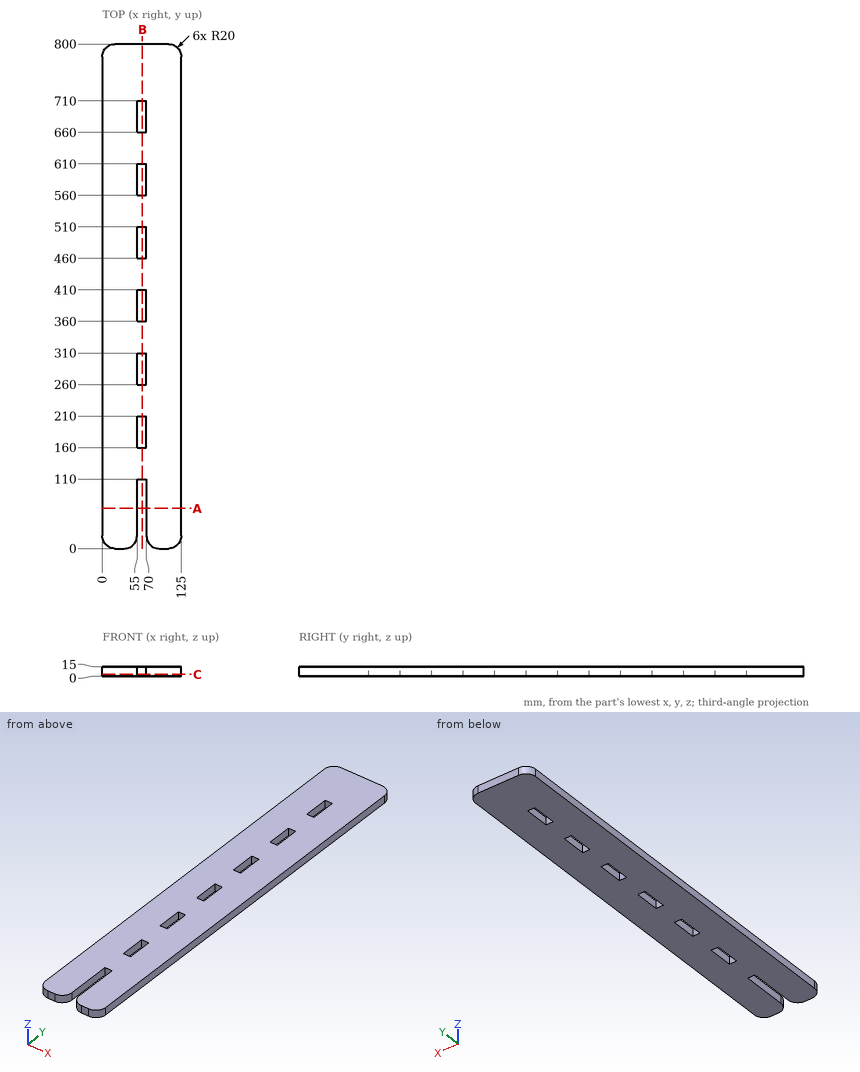
Design review of the part shown in the three views and the two pictorial views. Dimensions are in mm from the part's minimum x, y and z. Round coordinates to 2 decimals unless told otherwise and drop trailing zeros. Write each loop counter-clockwise with the first axis right and the second up, starting at its lowest first coordinate (ties: lowest second). Pieces come first, ordered by that corner, then holes. Notation, with made-up numbers: (-36.5, 12.25) -> (-29.5, 12.25) arc R16 cw to (-29.5, 20.25) -> close; hole circle Ø7 at (36.25, -6). An arc over 180 degrees is marked (long way). One line per question, with ' | ' between items. Start each with the question number.
1) Wall thickness on line 1 along X through (y, z) = (385, 2); line 2 along Y through (x, z) = (19, 5.5); line 3 along Y through (x, z) = (115, 14.25): over which ranges is each line inside the solid? List them lowest first.
2) Add section A-A (y = 63.5). Write out the cut boundary in (x, z), and give its area (3 significant figures).
3) Add section B-B (x = 63.5). Write out the cut boundary in (y, z).
4) For pin 1 Ø2 at (y, z) = (655, 5) entering from -X; pin 2 Ø7.5 at (x, z) = (63.5, 9) entering from -Y, all flat-tipped, find the tip position at first contact; note any pin that passes through.
5) Add section C-C (z = 2.75). Count the separate pieces of the cut face and the enclosed holes in it, and give its area (3 significant figures).
Reported:
1) line 1: x = 0 to 55, 70 to 125 | line 2: y = 0.03 to 799.97 | line 3: y = 2.68 to 797.32
2) outline: (0, 0) -> (55, 0) -> (55, 15) -> (0, 15) -> close; (70, 0) -> (125, 0) -> (125, 15) -> (70, 15) -> close | area: 1,650 mm²
3) outline: (110, 0) -> (160, 0) -> (160, 15) -> (110, 15) -> close; (210, 0) -> (260, 0) -> (260, 15) -> (210, 15) -> close; (310, 0) -> (360, 0) -> (360, 15) -> (310, 15) -> close; (410, 0) -> (460, 0) -> (460, 15) -> (410, 15) -> close; (510, 0) -> (560, 0) -> (560, 15) -> (510, 15) -> close; (610, 0) -> (660, 0) -> (660, 15) -> (610, 15) -> close; (710, 0) -> (800, 0) -> (800, 15) -> (710, 15) -> close
4) pin 1: stops at x = 0 | pin 2: stops at y = 110
5) separate pieces: 1 | enclosed holes: 6 | area: 93,300 mm²
